Read the model definition and answer for the solid it produces. Units are mm, in the model's axes. A direction names the side the tool comes from. Give positions to 0.01 mm unless a question says otherwise; leave off trailing zeros. Order: outer loops, then holes, each group sorted by start corner. A loop starts at its lowest first (then second) coordinate and runs counter-clockwise, first axis right, second up. Notation, with made-up numbers: M -13,24.5 L 8,24.5 A14 cw 8,30.5 Z; hole C -39,2.25 d11. An arc over 180 degrees is marked long. One line per item, written item: value.
from build123d import *

# Parameters (mm, degrees)
SKETCH1_W           = 275
SKETCH1_H           = 33
BOSS_EXTRUDE1_DEPTH = 12
CUT_EXTRUDE1_REACH  = 141.005
SKETCH2_R           = 11
SKETCH2_R_2         = 2.5
CUT_EXTRUDE2_REACH  = 141.005
SKETCH3_R           = 4
CUT_EXTRUDE3_REACH  = 143.913
SKETCH4_R           = 3


with BuildPart() as part:
    # Sketch1 → Boss-Extrude1 (new body)
    with BuildSketch(Plane.XY):
        Rectangle(SKETCH1_W, SKETCH1_H)
    extrude(amount=BOSS_EXTRUDE1_DEPTH)

    # Sketch2 → Cut-Extrude1 (cut, up to next)
    with BuildSketch(Plane.XY.offset(12), mode=Mode.PRIVATE) as cut_extrude1_sk1:
        with Locations((0, 1)):
            Circle(SKETCH2_R)
    cut_extrude1_tool1 = extrude(cut_extrude1_sk1.sketch, amount=-CUT_EXTRUDE1_REACH, mode=Mode.PRIVATE) & part.part
    # Sketch2 → Cut-Extrude1 (cut, up to next)
    with BuildSketch(Plane.XY.offset(12), mode=Mode.PRIVATE) as cut_extrude1_sk2:
        with Locations((-16.5, 1)):
            Circle(SKETCH2_R_2)
    cut_extrude1_tool2 = extrude(cut_extrude1_sk2.sketch, amount=-CUT_EXTRUDE1_REACH, mode=Mode.PRIVATE) & part.part
    # Sketch2 → Cut-Extrude1 (cut, up to next)
    with BuildSketch(Plane.XY.offset(12), mode=Mode.PRIVATE) as cut_extrude1_sk3:
        with Locations((16.5, 1)):
            Circle(SKETCH2_R_2)
    cut_extrude1_tool3 = extrude(cut_extrude1_sk3.sketch, amount=-CUT_EXTRUDE1_REACH, mode=Mode.PRIVATE) & part.part
    add(cut_extrude1_tool1.solids().sort_by_distance((0, 1, 12))[0], mode=Mode.SUBTRACT)
    add(cut_extrude1_tool2.solids().sort_by_distance((-16.5, 1, 12))[0], mode=Mode.SUBTRACT)
    add(cut_extrude1_tool3.solids().sort_by_distance((16.5, 1, 12))[0], mode=Mode.SUBTRACT)

    # Sketch3 → Cut-Extrude2 (cut, up to next)
    with BuildSketch(Plane.XY.offset(12), mode=Mode.PRIVATE) as cut_extrude2_sk1:
        with Locations((-100, 6.5)):
            Circle(SKETCH3_R)
    cut_extrude2_tool1 = extrude(cut_extrude2_sk1.sketch, amount=-CUT_EXTRUDE2_REACH, mode=Mode.PRIVATE) & part.part
    # Sketch3 → Cut-Extrude2 (cut, up to next)
    with BuildSketch(Plane.XY.offset(12), mode=Mode.PRIVATE) as cut_extrude2_sk2:
        with Locations((-50, 6.5)):
            Circle(SKETCH3_R)
    cut_extrude2_tool2 = extrude(cut_extrude2_sk2.sketch, amount=-CUT_EXTRUDE2_REACH, mode=Mode.PRIVATE) & part.part
    # Sketch3 → Cut-Extrude2 (cut, up to next)
    with BuildSketch(Plane.XY.offset(12), mode=Mode.PRIVATE) as cut_extrude2_sk3:
        with Locations((50, 6.5)):
            Circle(SKETCH3_R)
    cut_extrude2_tool3 = extrude(cut_extrude2_sk3.sketch, amount=-CUT_EXTRUDE2_REACH, mode=Mode.PRIVATE) & part.part
    # Sketch3 → Cut-Extrude2 (cut, up to next)
    with BuildSketch(Plane.XY.offset(12), mode=Mode.PRIVATE) as cut_extrude2_sk4:
        with Locations((100, 6.5)):
            Circle(SKETCH3_R)
    cut_extrude2_tool4 = extrude(cut_extrude2_sk4.sketch, amount=-CUT_EXTRUDE2_REACH, mode=Mode.PRIVATE) & part.part
    add(cut_extrude2_tool1.solids().sort_by_distance((-100, 6.5, 12))[0], mode=Mode.SUBTRACT)
    add(cut_extrude2_tool2.solids().sort_by_distance((-50, 6.5, 12))[0], mode=Mode.SUBTRACT)
    add(cut_extrude2_tool3.solids().sort_by_distance((50, 6.5, 12))[0], mode=Mode.SUBTRACT)
    add(cut_extrude2_tool4.solids().sort_by_distance((100, 6.5, 12))[0], mode=Mode.SUBTRACT)

    # Sketch4 → Cut-Extrude3 (cut, up to next)
    with BuildSketch(Plane(origin=(0, 16.5, 0), x_dir=(1, 0, 0), z_dir=(0, 1, 0)), mode=Mode.PRIVATE) as cut_extrude3_sk1:
        with Locations(Location((-100, -6, 0), (0, 0, 270))):
            Circle(SKETCH4_R)
    cut_extrude3_tool1 = extrude(cut_extrude3_sk1.sketch, amount=-CUT_EXTRUDE3_REACH, mode=Mode.PRIVATE) & part.part
    # Sketch4 → Cut-Extrude3 (cut, up to next)
    with BuildSketch(Plane(origin=(0, 16.5, 0), x_dir=(1, 0, 0), z_dir=(0, 1, 0)), mode=Mode.PRIVATE) as cut_extrude3_sk2:
        with Locations(Location((-50, -6, 0), (0, 0, 270))):
            Circle(SKETCH4_R)
    cut_extrude3_tool2 = extrude(cut_extrude3_sk2.sketch, amount=-CUT_EXTRUDE3_REACH, mode=Mode.PRIVATE) & part.part
    # Sketch4 → Cut-Extrude3 (cut, up to next)
    with BuildSketch(Plane(origin=(0, 16.5, 0), x_dir=(1, 0, 0), z_dir=(0, 1, 0)), mode=Mode.PRIVATE) as cut_extrude3_sk3:
        with Locations(Location((50, -6, 0), (0, 0, 270))):
            Circle(SKETCH4_R)
    cut_extrude3_tool3 = extrude(cut_extrude3_sk3.sketch, amount=-CUT_EXTRUDE3_REACH, mode=Mode.PRIVATE) & part.part
    # Sketch4 → Cut-Extrude3 (cut, up to next)
    with BuildSketch(Plane(origin=(0, 16.5, 0), x_dir=(1, 0, 0), z_dir=(0, 1, 0)), mode=Mode.PRIVATE) as cut_extrude3_sk4:
        with Locations(Location((100, -6, 0), (0, 0, 270))):
            Circle(SKETCH4_R)
    cut_extrude3_tool4 = extrude(cut_extrude3_sk4.sketch, amount=-CUT_EXTRUDE3_REACH, mode=Mode.PRIVATE) & part.part
    add(cut_extrude3_tool1.solids().sort_by_distance((-100, 16.5, 6))[0], mode=Mode.SUBTRACT)
    add(cut_extrude3_tool2.solids().sort_by_distance((-50, 16.5, 6))[0], mode=Mode.SUBTRACT)
    add(cut_extrude3_tool3.solids().sort_by_distance((50, 16.5, 6))[0], mode=Mode.SUBTRACT)
    add(cut_extrude3_tool4.solids().sort_by_distance((100, 16.5, 6))[0], mode=Mode.SUBTRACT)


solid = part.part
1) Which of the six approach directions +Z, -Z, +X, -X, +Y, -Y give full straight-line access (tool end or side, diameter ignored) to faces 4 (the face through (-2, -11, 0)), 5 (the face through (-101.15, 12.87, 8.77))?
Reported:
face 4: -Z, +X, -X, +Y, -Y
face 5: +Y
2) Each of these flat-tipped pins is pushed along its axis until it touches: pin 1 Ø13 at (x, y) = (-100, 6.5) entering from +Z; pin 2 Ø17.5 at (x, y) = (0, 1) entering from -Z. Where does it stop, or does it pass through?
Reported:
pin 1: stops at z = 12
pin 2: passes through
3) Find section B-B, the plane x = 50. Write down the section's boundary in (y, z), plus the area to 3 significant figures.
Reported:
outline: M -16.5,0 L 2.5,0 L 2.5,12 L -16.5,12 Z; M 10.5,0 L 16.5,0 L 16.5,3 L 10.5,3 Z; M 10.5,9 L 16.5,9 L 16.5,12 L 10.5,12 Z
area: 264 mm^2
4) Determine the mould class of faces 1 (the face through (50.9, 12.87, 8.86)), 2 (the face through (-2, -11, 12)), 3 (the face through (-2, 16.5, 6)) for opening direction Z: +Z half, -Z half, draft (parallel to the pull), parting line (faces both ways), or undercut.
Reported:
face 1: undercut
face 2: +Z half
face 3: draft
5) Find section C-C, the plane y = 6.5. Write down the section's boundary in (x, z).
Reported:
outline: M -137.5,0 L -104,0 L -104,12 L -137.5,12 Z; M -96,0 L -54,0 L -54,12 L -96,12 Z; M -46,0 L -9.53,0 L -9.53,12 L -46,12 Z; M 9.53,0 L 46,0 L 46,12 L 9.53,12 Z; M 54,0 L 96,0 L 96,12 L 54,12 Z; M 104,0 L 137.5,0 L 137.5,12 L 104,12 Z
6) Find section A-A, the plane x = 16.5. Write down the section's boundary in (y, z).
Reported:
outline: M -16.5,0 L -1.5,0 L -1.5,12 L -16.5,12 Z; M 3.5,0 L 16.5,0 L 16.5,12 L 3.5,12 Z
7) Consider probe 1 along X at (y, z) = (12.75, 6); probe 2 along Z at (x, y) = (-100, 14); probe 3 along X at (y, z) = (8, 9.5). Determine where each line is inside the solid, lowest interval first.
Reported:
probe 1: x = -137.5 to -103, -97 to -53, -47 to 47, 53 to 97, 103 to 137.5
probe 2: z = 0 to 3, 9 to 12
probe 3: x = -137.5 to -103.71, -96.29 to -53.71, -46.29 to -8.49, 8.49 to 46.29, 53.71 to 96.29, 103.71 to 137.5
